Input: part model. Units: mm. Frame: model coordinates. A direction names the side the tool comes from. Coordinates: 2 decimals unless noted, no trailing zeros. Write each loop counter-clockwise with the first axis right and the second up, starting at its lowest first coordinate (ties: lowest second). Pieces come first, ordered by that corner, then holes.
1) Section query A-A (y = 10). Output: boundary loops of the cut face in (x, z), then the cut area to 3 significant figures.
2) Section query D-D (y = 5). Output: boundary loops of the cut face in (x, z).
3) Pin query (flat end, axial travel): pin 1 Ø5 at (x, y) = (28, 6) entering from -Z; pin 2 Ø3.5 at (x, y) = (44.75, 5) entering from -Z; pin 3 Ø10 at (y, z) = (13, 19.5) entering from -X; pin 4 Ø12 at (x, y) = (20.5, 5) entering from +Z. Return the tip coordinate at first contact, or that it passes through.
4) Draft query along Y for faces 6 (the cylindrical face through (43.25, 15.05, 39.01)), 7 (the flat face through (-6, 10, 39)), 8 (the flat face through (20, 20, 22)), 9 (the cylindrical face through (43.25, 5.05, 39.01)). Return one class per face: pulls with the +Y half, pulls with the -Y half, needs draft (parallel to the pull), parting line crosses it, or undercut.
5) Line query: L1, parallel to Y at x = 44.75, z = 38.85; L2, parallel to Z at x = 7.5, y = 16.75; L3, parallel to X at y = 8.75, z = 13. Output: solid intervals per line, ascending.
6) Set-up query: faces 1 (the flat face through (-6, 2, 39)), 2 (the flat face through (0, 10, 19)), 3 (the flat face through (40, 10, 19)), 4 (the flat face through (20, 10, 45)), 5 (the flat face through (43, 10, 40)). Return all of +Z, -Z, +X, -X, +Y, -Y with unobstructed straight access to the full face (end or side cutting, diameter ignored); none if empty.
7) Section query C-C (z = 33). Output: boundary loops of the cut face in (x, y), then the cut area to 3 significant figures.
8) Section query B-B (x = 35). Output: boundary loops of the cut face in (y, z).
from build123d import *

# Parameters (mm, degrees)
ESQUISSE1_W             = 40
ESQUISSE1_H             = 20
BOSS_EXTRU_1_DEPTH      = 45
ESQUISSE2_R             = 4
BOSS_EXTRU_2_DEPTH      = 3
ESQUISSE3_W             = 2
ESQUISSE3_H             = 20
BOSS_EXTRU_3_DEPTH      = 6
ESQUISSE4_W             = 2
ESQUISSE4_H             = 20
BOSS_EXTRU_4_DEPTH      = 6
ESQUISSE5_R             = 1.5
ENL_V_MAT_EXTRU_1_DEPTH = 6


with BuildPart() as part:
    # Esquisse1 → Boss.-Extru.1 (new body)
    with BuildSketch(Plane.XY):
        with Locations((20, 10)):
            Rectangle(ESQUISSE1_W, ESQUISSE1_H)
    extrude(amount=BOSS_EXTRU_1_DEPTH)

    # Esquisse2 → Boss.-Extru.2 (add)
    with BuildSketch(Plane.XY.offset(45)):
        with Locations(Location((5, 10, 0), (0, 0, 180))):
            Circle(ESQUISSE2_R)
        with Locations(Location((35, 10, 0), (0, 0, 180))):
            Circle(ESQUISSE2_R)
    extrude(amount=BOSS_EXTRU_2_DEPTH)

    # Esquisse3 → Boss.-Extru.3 (add)
    with BuildSketch(Plane.ZY):
        with Locations((39, 10)):
            Rectangle(ESQUISSE3_W, ESQUISSE3_H)
    extrude(amount=BOSS_EXTRU_3_DEPTH)

    # Esquisse4 → Boss.-Extru.4 (add)
    with BuildSketch(Plane(origin=(40, 0, 0), x_dir=(0, 0, -1), z_dir=(1, 0, 0))):
        with Locations((-39, 10)):
            Rectangle(ESQUISSE4_W, ESQUISSE4_H)
    extrude(amount=BOSS_EXTRU_4_DEPTH)

    # Esquisse5 → Enlèv. mat.-Extru.1 (cut)
    with BuildSketch(Plane.XY.offset(40)):
        with Locations((-4.75, 15)):
            Circle(ESQUISSE5_R)
        with Locations((-4.75, 5)):
            Circle(ESQUISSE5_R)
        with Locations((44.75, 15)):
            Circle(ESQUISSE5_R)
        with Locations((44.75, 5)):
            Circle(ESQUISSE5_R)
    extrude(amount=-ENL_V_MAT_EXTRU_1_DEPTH, mode=Mode.SUBTRACT)


solid = part.part
Answer:
1. outline: (-6, 38) - (0, 38) - (0, 0) - (40, 0) - (40, 38) - (46, 38) - (46, 40) - (40, 40) - (40, 45) - (39, 45) - (39, 48) - (31, 48) - (31, 45) - (9, 45) - (9, 48) - (1, 48) - (1, 45) - (0, 45) - (0, 40) - (-6, 40) - close
1. area: 1,870 mm2
2. outline: (-3.25, 38) - (0, 38) - (0, 0) - (40, 0) - (40, 38) - (43.25, 38) - (43.25, 40) - (40, 40) - (40, 45) - (0, 45) - (0, 40) - (-3.25, 40) - close
3. pin 1: stops at z = 0
3. pin 2: stops at z = 38
3. pin 3: stops at x = 0
3. pin 4: stops at z = 45
4. face 6: undercut
4. face 7: needs draft
4. face 8: pulls with the +Y half
4. face 9: undercut
5. L1: y = 0 to 3.5, 6.5 to 13.5, 16.5 to 20
5. L2: z = 0 to 45
5. L3: x = 0 to 40
6. face 1: +Z, -Z, -X, +Y, -Y
6. face 2: -Z, -X, +Y, -Y
6. face 3: -Z, +X, +Y, -Y
6. face 4: +Z
6. face 5: +Z, +X, +Y, -Y
7. outline: (0, 0) - (40, 0) - (40, 20) - (0, 20) - close
7. area: 800 mm2
8. outline: (0, 0) - (20, 0) - (20, 45) - (14, 45) - (14, 48) - (6, 48) - (6, 45) - (0, 45) - close
